from build123d import *

# Parameters (mm, degrees)
EXTRUDE_1_OUTLINE_R     = 8.5
EXTRUDE_1_OUTLINE_R_2   = 2
EXTRUDE_1_DEPTH         = 3
SKETCH_2_5_R            = 8.5
SKETCH_2_5_R_2          = 1.5
EXTRUDE_3_DEPTH         = 2
CUT_EXTRUDE_START       = -3
CUT_EXTRUDE_1_OUTLINE_R = 1.5
CUT_EXTRUDE_1_DEPTH     = 3
SKETCH_14_R             = 21
SKETCH_14_R_2           = 11
CUT_EXTRUDE_2_DEPTH     = 0.5
SKETCH_15_R             = 9.5
SKETCH_15_R_2           = 8.5
EXTRUDE_4_DEPTH         = 0.5
SKETCH_15_3_R           = 11
SKETCH_15_3_R_2         = 9.5
CUT_EXTRUDE_3_DEPTH     = 0.5
SKETCH_17_R             = 3.5
CUT_EXTRUDE_4_DEPTH     = 1.5
HOLE_WIZARD_M2_1_D      = 1.6
CHAMFER_1_SIZE          = 0.5
CHAMFER_2_SIZE          = 1
CHAMFER_3_SIZE          = 1
CHAMFER_4_SIZE          = 1.5


# Read off the part's stored shape, not the designer's step: 凸台-拉伸1, 切除-拉伸1
with BuildPart() as part:
    # 凸台-拉伸1 outline → 凸台-拉伸1 (new body)
    with BuildSketch(Plane(origin=(0, 0, 0), x_dir=(1, 0, 0), z_dir=(0, 1, 0))):
        with BuildLine():
            add(Edge.make_bspline(
                [(-17.166812063, -88.021637563), (-38.974423907, -66.214025718), (-38.974423907, 14.170750592)],
                knots=[0, 0, 0, 1, 1, 1], degree=2))
            ThreePointArc((-17.166812063, -88.021637563), (-7.974423908, -91.829249408), (1.217964248, -88.021637563))
            add(Edge.make_bspline(
                [(1.217964248, -88.021637563), (23.025576093, -66.214025718), (23.025576093, 14.170750592)],
                knots=[0, 0, 0, 1, 1, 1], degree=2))
            Line((23.025576093, 14.170750592), (23.025576093, 34.170750592))
            Line((23.025576093, 34.170750592), (-38.974423907, 34.170750592))
            Line((-38.974423907, 34.170750592), (-38.974423907, 14.170750592))
        make_face()
        with Locations((-7.974423907, -78.829249408)):
            Circle(EXTRUDE_1_OUTLINE_R, mode=Mode.SUBTRACT)
        with Locations((-28.974423907, 29.170750592)):
            Circle(EXTRUDE_1_OUTLINE_R_2, mode=Mode.SUBTRACT)
        with Locations((-7.974423907, 29.170750592)):
            Circle(EXTRUDE_1_OUTLINE_R_2, mode=Mode.SUBTRACT)
        with Locations((13.025576093, 29.170750592)):
            Circle(EXTRUDE_1_OUTLINE_R_2, mode=Mode.SUBTRACT)
    extrude(amount=EXTRUDE_1_DEPTH)

    # 草图2<5> → 凸台-拉伸3 (add)
    with BuildSketch(Plane(origin=(0, 0, 0), x_dir=(1, 0, 0), z_dir=(0, 1, 0))):
        with Locations(Location((-7.974423907, -78.829249408, 0), (0, 0, 270))):
            Circle(SKETCH_2_5_R)
        with Locations(Location((-7.974423907, -78.829249408, 0), (0, 0, 270))):
            Circle(SKETCH_2_5_R_2, mode=Mode.SUBTRACT)
        with Locations(Location((-7.974423907, -83.829249408, 0), (0, 0, 270))):
            Circle(SKETCH_2_5_R_2, mode=Mode.SUBTRACT)
        with Locations(Location((-12.304550926, -76.329249408, 0), (0, 0, 270))):
            Circle(SKETCH_2_5_R_2, mode=Mode.SUBTRACT)
        with Locations(Location((-3.644296889, -76.329249408, 0), (0, 0, 270))):
            Circle(SKETCH_2_5_R_2, mode=Mode.SUBTRACT)
    extrude(amount=EXTRUDE_3_DEPTH)

    # 切除-拉伸1 outline → 切除-拉伸1 (cut)
    with BuildSketch(Plane(origin=(0, 3, 0), x_dir=(1, 0, 0), z_dir=(0, 1, 0)).offset(CUT_EXTRUDE_START)):
        with Locations((-20.474423907, -23.829249408)):
            Circle(CUT_EXTRUDE_1_OUTLINE_R)
        with Locations((-7.974423907, -43.829249408)):
            Circle(CUT_EXTRUDE_1_OUTLINE_R)
        with Locations((4.525576093, -23.829249408)):
            Circle(CUT_EXTRUDE_1_OUTLINE_R)
        with Locations((-35.966826399, 11.170789443)):
            Circle(CUT_EXTRUDE_1_OUTLINE_R)
        with BuildLine():
            ThreePointArc((20.028398358, 12.670753252), (20.021777301, 12.670755407), (20.015156318, 12.670786788))
            ThreePointArc((20.015156318, 12.670786788), (20.014179778, 9.670794253), (20.028398358, 12.670753252))
        make_face()
    extrude(amount=CUT_EXTRUDE_1_DEPTH, mode=Mode.SUBTRACT)

    # 草图14 → 切除-拉伸2 (cut)
    with BuildSketch(Plane(origin=(0, 3, 0), x_dir=(1, 0, 0), z_dir=(0, 1, 0))):
        with Locations((-7.974423907, -78.829249408)):
            Circle(SKETCH_14_R)
        with Locations(Location((-7.974423907, -78.829249408, 0), (0, 0, 270))):
            Circle(SKETCH_14_R_2, mode=Mode.SUBTRACT)
    extrude(amount=-CUT_EXTRUDE_2_DEPTH, mode=Mode.SUBTRACT)

    # 草图15 → 凸台-拉伸4 (add)
    with BuildSketch(Plane(origin=(0, 3, 0), x_dir=(1, 0, 0), z_dir=(0, 1, 0))):
        with Locations(Location((-7.974423907, -78.829249408, 0), (0, 0, 270))):
            Circle(SKETCH_15_R)
        with Locations(Location((-7.974423907, -78.829249408, 0), (0, 0, 270))):
            Circle(SKETCH_15_R_2, mode=Mode.SUBTRACT)
    extrude(amount=EXTRUDE_4_DEPTH)

    # 草图15<3> → 切除-拉伸3 (cut)
    with BuildSketch(Plane(origin=(0, 3, 0), x_dir=(1, 0, 0), z_dir=(0, 1, 0))):
        with Locations((-7.974423907, -78.829249408)):
            Circle(SKETCH_15_3_R)
        with Locations(Location((-7.974423907, -78.829249408, 0), (0, 0, 270))):
            Circle(SKETCH_15_3_R_2, mode=Mode.SUBTRACT)
    extrude(amount=-CUT_EXTRUDE_3_DEPTH, mode=Mode.SUBTRACT)

    # 草图17 → 切除-拉伸4 (cut)
    with BuildSketch(Plane(origin=(0, 3, 0), x_dir=(1, 0, 0), z_dir=(0, 1, 0))):
        with BuildLine():
            Line((13.025576092, 14.170750422), (13.025576093, 24.170750592))
            Line((13.025576093, 24.170750592), (-28.974423907, 24.170750592))
            Line((-28.974423907, 24.170750592), (-28.974423907, 14.170750592))
            add(Edge.make_bspline(
                [(-28.974423907, 14.170750592), (-28.974423907, 13.311861342), (-28.970577127, 11.586194366), (-28.947516149, 8.198019857), (-28.889914894, 4.037728889), (-28.774892402, -0.820742579), (-28.560545128, -7.124589729), (-28.178715271, -14.674765284), (-27.540114076, -23.204861593), (-26.723596489, -31.200556861), (-25.89763435, -37.41453686), (-25.151910121, -42.11313709), (-24.550677966, -45.500866022), (-24.016057668, -48.206887938), (-23.56719588, -50.307521536), (-23.33835214, -51.325314161), (-23.220255995, -51.837313496)],
                knots=[0.495235673, 0.495235673, 0.495235673, 0.495235673, 0.495300523, 0.495365373, 0.495495073, 0.495624773, 0.495754473, 0.496013874, 0.496273274, 0.496532675, 0.496792075, 0.496921775, 0.497051475, 0.497181176, 0.497246026, 0.497310876, 0.497310876, 0.497310876, 0.497310876], degree=3))
            ThreePointArc((-23.220255995, -51.837313496), (-17.53895703, -49.341629884), (-11.474423907, -48.027463761))
            Line((-11.474423907, -48.027463761), (-11.474423907, -43.829249408))
            ThreePointArc((-11.474423907, -43.829249408), (-7.974423907, -40.329249408), (-4.474423907, -43.829249408))
            Line((-4.474423907, -43.829249408), (-4.474423907, -48.027463766))
            ThreePointArc((-4.474423907, -48.027463766), (1.590109217, -49.341629893), (7.271408173, -51.837313525))
            add(Edge.make_bspline(
                [(7.271408173, -51.837313525), (7.389504318, -51.325314191), (7.618348058, -50.307521568), (8.067209846, -48.206887974), (8.601830143, -45.500866064), (9.203062298, -42.113137138), (9.948786527, -37.414536918), (10.774748665, -31.200556932), (11.591266253, -23.20486168), (12.22986745, -14.674765389), (12.611697308, -7.124589851), (12.826044583, -0.820742715), (12.941067076, 4.037728742), (12.998668332, 8.198019701), (13.021729311, 11.586194202), (13.025576092, 13.311861174), (13.025576092, 14.170750422)],
                knots=[0.502689124, 0.502689124, 0.502689124, 0.502689124, 0.502753974, 0.502818824, 0.502948525, 0.503078225, 0.503207925, 0.503467325, 0.503726726, 0.503986126, 0.504245527, 0.504375227, 0.504504927, 0.504634627, 0.504699477, 0.504764327, 0.504764327, 0.504764327, 0.504764327], degree=3))
        make_face()
        with Locations(Location((-20.474423907, -23.829249408, 0), (0, 0, 270))):
            Circle(SKETCH_17_R, mode=Mode.SUBTRACT)
        with Locations(Location((4.525576093, -23.829249408, 0), (0, 0, 270))):
            Circle(SKETCH_17_R, mode=Mode.SUBTRACT)
    extrude(amount=-CUT_EXTRUDE_4_DEPTH, mode=Mode.SUBTRACT)

    # M2 螺纹孔1 (through all)
    with Locations(Plane(origin=(-14.974423907, 0, -21.170750592), x_dir=(0, 0, -1), z_dir=(0, -1, 0))):
        with Locations((0, 0), (0, 16)):
            Hole(HOLE_WIZARD_M2_1_D / 2)

    # 倒角1
    chamfer_1_edges = [part.edges().sort_by_distance(p)[0] for p in [
        (-7.974423907, 3, 57.829249408),
    ]]
    chamfer(chamfer_1_edges, length=CHAMFER_1_SIZE - 0.0001)  # a hair under: the kernel refuses the full size

    # 倒角2
    chamfer_2_edges = [part.edges().sort_by_distance(p)[0] for p in [
        (-38.974423907, 0, -24.170750592),
        (23.025576093, 0, -24.170750592),
        (-7.974423907, 0, 91.829249408),
    ]]
    chamfer(chamfer_2_edges, length=CHAMFER_2_SIZE)

    # 倒角3
    chamfer_3_edges = [part.edges().sort_by_distance(p)[0] for p in [
        (-7.974423907, 2.5, 69.329249408),
    ]]
    chamfer(chamfer_3_edges, length=CHAMFER_3_SIZE - 0.0001)  # a hair under: the kernel refuses the full size

    # 倒角4
    chamfer_4_edges = [part.edges().sort_by_distance(p)[0] for p in [
        (1.590109217, 1.5, 49.341629893),
    ]]
    chamfer(chamfer_4_edges, length=CHAMFER_4_SIZE - 0.0001)  # a hair under: the kernel refuses the full size
    chamfer_4_2_edges = [part.edges().sort_by_distance(p)[0] for p in [
        (-4.474423907, 1.5, 45.173805289),
        (-7.974423907, 1.5, 40.329249408),
        (-11.474423907, 1.5, 45.928356584),
    ]]
    chamfer(chamfer_4_2_edges, length=CHAMFER_4_SIZE - 0.0001)  # a hair under: the kernel refuses the full size
    chamfer_4_3_edges = [part.edges().sort_by_distance(p)[0] for p in [
        (-18.256270706, 1.5, 49.584016882),
    ]]
    chamfer(chamfer_4_3_edges, length=CHAMFER_4_SIZE - 0.0001)  # a hair under: the kernel refuses the full size
    chamfer_4_4_edges = [part.edges().sort_by_distance(p)[0] for p in [
        (-27.599295062, 1.5, 22.087266062),
        (-28.974423907, 1.5, -19.170750592),
    ]]
    chamfer(chamfer_4_4_edges, length=CHAMFER_4_SIZE - 0.0001)  # a hair under: the kernel refuses the full size
    chamfer_4_5_edges = [part.edges().sort_by_distance(p)[0] for p in [
        (-7.224473907, 1.5, -24.170750592),
    ]]
    chamfer(chamfer_4_5_edges, length=CHAMFER_4_SIZE - 0.0001)  # a hair under: the kernel refuses the full size
    chamfer_4_6_edges = [part.edges().sort_by_distance(p)[0] for p in [
        (13.025576092, 1.5, -18.420800507),
        (11.65044724, 1.5, 22.087266148),
    ]]
    chamfer(chamfer_4_6_edges, length=CHAMFER_4_SIZE - 0.0001)  # a hair under: the kernel refuses the full size
    chamfer_4_7_edges = [part.edges().sort_by_distance(p)[0] for p in [
        (-20.474423907, 1.5, 20.329249408),
    ]]
    chamfer(chamfer_4_7_edges, length=CHAMFER_4_SIZE - 0.0001)  # a hair under: the kernel refuses the full size
    chamfer_4_8_edges = [part.edges().sort_by_distance(p)[0] for p in [
        (4.525576093, 1.5, 20.329249408),
    ]]
    chamfer(chamfer_4_8_edges, length=CHAMFER_4_SIZE - 0.0001)  # a hair under: the kernel refuses the full size


solid = part.part
The listing builds one solid part. Answer for the finished solid, in the listing's coordinates (mm). A direction names the side the tool comes from. Give positions to 0.01 mm unless a question says otherwise; leave off trailing zeros.
Item 1: Flat-ended cylindrical pins translate along their axes: P1, Ø5, axis at x = -12.3, z = 76.33, coming from the +Y side; P2, Ø1, axis at x = 1.03, z = -21.17, coming from the -Y side; P3, Ø3.5, axis at x = -20.47, z = 23.83, coming from the +Y side; P4, Ø1.5, axis at x = -6.5, z = 17.5, coming from the +Y side. Find the tip coordinate at first contact, or state that the pin passes through.
Item 2: Determine the mould class of faces 3 (the flat face through (3.8, 3, 25.34)), 4 (the cylindrical face through (-12.24, 0.99, 74.83)), 5 (the cylindrical face through (-8.235, 1.479, -31.154)) for opening direction X: released by +X, released by -X, zero draft, split by the parting line, or undercut.
Item 3: Find the intervals of material crossed by line 1 along Y through (x, z) = (-32, 15); line 2 along X through (y, z) = (2.05, 44); line 3 along X through (y, z) = (0.55, 23.5), in increasing order.
Item 4: Which of the six approach directions +Z, -Z, +X, -X, +Y, -Y give full straight-line access (tool end or side, diameter ignored) to faces 1 (the cylindrical face through (-30.45, 1.48, -30.52)), 2 (the flat face through (-8, 2.5, 67))?
Completed:
1. P1: stops at y = 2
1. P2: passes through
1. P3: stops at y = 3
1. P4: stops at y = 1.5
2. face 3: zero draft
2. face 4: undercut
2. face 5: undercut
3. line 1: y = 0 to 3
3. line 2: x = -34.96 to -23.85, -12.42 to -9.46, -6.48 to -3.52, 7.9 to 19.02
3. line 3: x = -37.06 to -21.94, -19.01 to 3.06, 5.99 to 21.11
4. face 1: +Y, -Y
4. face 2: +Y
